```python
from build123d import *

# Parameters (mm, degrees)
F0_R     = 2
F1_DEPTH = 39
F2_SIZE2 = 0.5
F2_SIZE  = 0.5
F3_R     = 3
F4_DEPTH = 3
F5_R     = 2.99999
F6_R     = 0.5
F7_DEPTH = 12.5


# Not quite as in the source:
# - a fillet or chamfer is up to 0.001 mm smaller than in the source, because OpenCascade refuses the exact size


with BuildPart() as f1:
    # F0 (on Top) → F1 (new body)
    with BuildSketch(Plane.XY):
        Circle(F0_R)
    extrude(amount=F1_DEPTH)

    # F2
    f2_edges = [f1.edges().sort_by_distance(p)[0] for p in [
        (-2, 0, 0),
    ]]
    chamfer(f2_edges, length=F2_SIZE, length2=F2_SIZE2)

    # F3 (on face) → F4 (join)
    with BuildSketch(Plane.XY.offset(39)):
        Circle(F3_R)
    extrude(amount=F4_DEPTH)

    # F5 (radius 3 in the source; OpenCascade refuses exactly that, so slightly less here)
    f5_edges = [f1.edges().sort_by_distance(p)[0] for p in [
        (-3, 0, 42),
    ]]
    fillet(f5_edges, radius=F5_R)

    # F6 (on Right) → F7 (cut, symmetric)
    with BuildSketch(Plane.YZ):
        with Locations((0, 2)):
            Circle(F6_R)
    extrude(amount=F7_DEPTH, both=True, mode=Mode.SUBTRACT)


solid = f1.part
```
Work out the finished part from the listing and answer in its coordinate system (mm). Give positions to 0.01 mm unless a question says otherwise; leave off trailing zeros. Loops run counter-clockwise (first coordinate to the right, second up) from the corner with the lowest first, then second, coordinate; pieces in that order, holes last. Notation, with made-up numbers: (-30, 75.5) -> (-13, 75.5) arc R23 ccw to (-13, 98.5) -> close; hole circle Ø11 at (88.25, 87). An arc over 180 degrees is marked (long way). Write item = value, one per line. Start each with the question number.
(1) Find section B-B on z = 37. Give the vertices of the cut face in (x, y), and give its area (3 significant figures).
(2) The mould has two halves that part along Z. Classify faces 1 (the flat face through (0, 0, 0)), 2 (the cylindrical face through (0.028, -0.065, 2.496)): +Z half, -Z half, draft (parallel to the pull), parting line (faces both ways), or undercut.
(3) Find section A-A on z = 2. Give the vertices of the cut face in (x, y).
(4) Find the intervals of material crossed by probe 1 along Z at (x, y) = (-0.1, 0); probe 2 along Z at (x, y) = (-0.6, 0); probe 3 along X at (y, z) = (-1, 3), in increasing order. Write a range as from..to.
(5) Given pin 1 Ø2 at (x, z) = (2, 29) entering from -Y; pin 2 Ø2 at (y, z) = (-0.5, 29) entering from +X; pin 3 Ø2 at (y, z) = (1, 34) entering from -X, each flat-ended and moving along its own axis, determine where each tip first touches the part or whether it passes through.
From the geometry:
q1.outline = circle Ø4 at (0, 0)
q1.area = 12.6 mm^2
q2.face_1 = -Z half
q2.face_2 = undercut
q3.outline = (-1.94, -0.5) arc R2 ccw to (1.94, -0.5) -> close; (-1.94, 0.5) -> (1.94, 0.5) arc R2 ccw to start
q4.probe_1 = 0..1.5, 2.5..42
q4.probe_2 = 0..1.5, 2.5..41.94
q4.probe_3 = -1.73..1.73
q5.pin_1 = -1.73
q5.pin_2 = 2
q5.pin_3 = -2
